Verification items for this drawing (mm, ordinates from the low corner). A direction names the side the tool comes from. Coordinates: 2 decimals unless noted, no trailing zeros. Order: outer loops, then holes, each group sorted by start corner. A loop starts at its lowest first (then second) coordinate and runs counter-clockwise, first axis right, second up. Notation, with made-up numbers: (55.25, 38.25) -> (59.25, 38.25) arc R4 cw to (59.25, 44.25) -> close; hole circle Ø11 at (-16, -31). An arc over 180 degrees is marked (long way). Write item = value, one per line. Start each with the question number.
1. Thickness scan on line 1 along Y through (x, z) = (13.97, 38.8); line 2 along Y through (x, z) = (13.5, 8); line 3 along X through (y, z) = (9, 4.5) (1 decimal). Record the ranges inside material, lowest first. Write a range as from..to.
2. Cross-section at A-A on x = 13.97. Record the cut outline in (y, z).
3. Set-up check for the marked faces 3 and 4: record each of +Z, -Z, +X, -X, +Y, -Y from which the full face is reachable in a straight line by a thin tool's end or side.
4. Cross-section at B-B on z = 36.5. Record the cut outline in (x, y).
5. Release check for a two-part mould opening along Y. For the marked faces 1 and 2 record: +Y half, -Y half, draft (parallel to the pull), parting line (faces both ways), or undercut.
6. Go/stop test with flat-tipped pins: P1, Ø5, axis at y = 3, z = 17, coming from the +X side; P2, Ø4, axis at x = 13, z = 22, coming from the +Y side; P3, Ø4, axis at x = 5, z = 17.5, coming from the +Y side. Record where each tip stops, or that it passes through.
7. Cross-section at C-C on z = 13. Record the cut outline in (x, y).
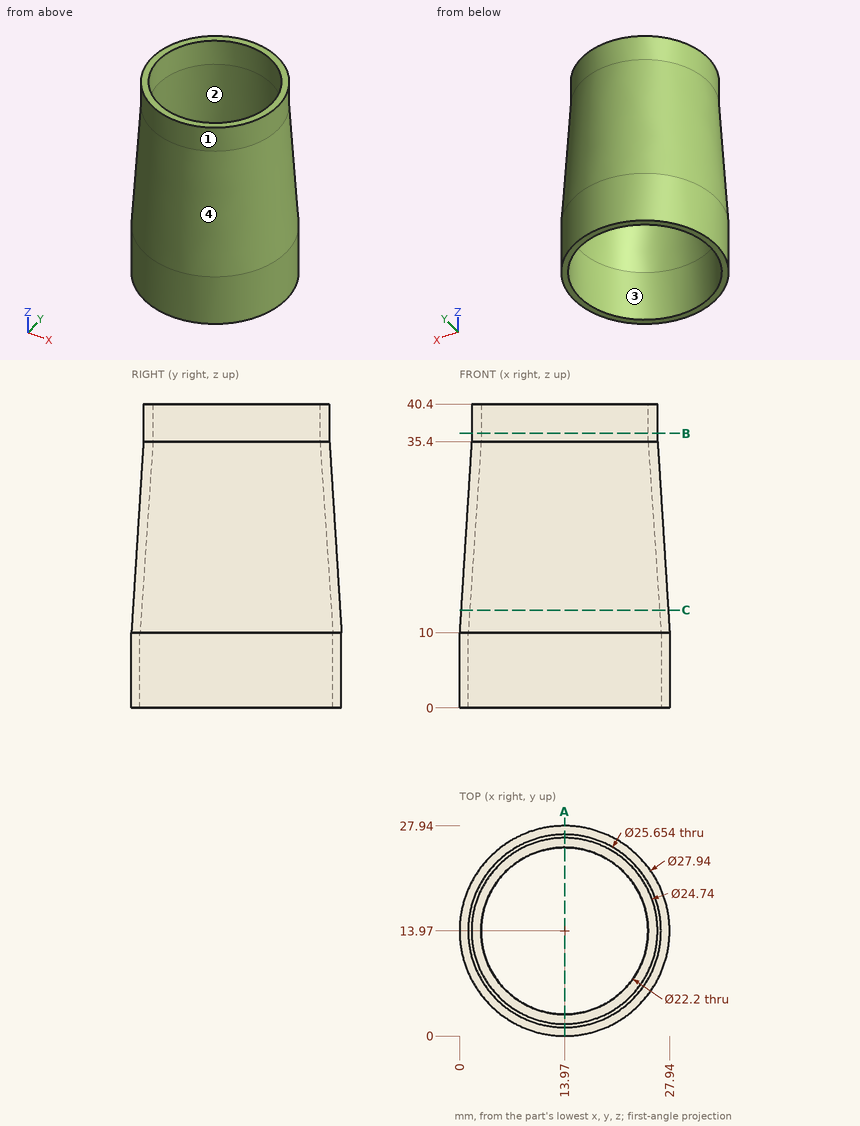
Worked out:
q1.line_1 = 1.6..2.87, 25.07..26.34
q1.line_2 = 0.01..1.15, 26.79..27.93
q1.line_3 = 0.9..2.1, 25.8..27
q2.outline = (0, 0) -> (1.14, 0) -> (1.14, 10) -> (2.87, 35.4) -> (2.87, 40.4) -> (1.6, 40.4) -> (1.6, 35.4) -> (0, 10) -> close; (25.07, 35.4) -> (26.8, 10) -> (26.8, 0) -> (27.94, 0) -> (27.94, 10) -> (26.34, 35.4) -> (26.34, 40.4) -> (25.07, 40.4) -> close
q3.face_3 = -Z
q3.face_4 = +Z
q4.outline = circle Ø24.74 at (13.97, 13.97); hole circle Ø22.2 at (13.97, 13.97)
q5.face_1 = parting line
q5.face_2 = undercut
q6.P1 = 24.53
q6.P2 = 27.3
q6.P3 = 25.54
q7.outline = circle Ø27.56 at (13.97, 13.97); hole circle Ø25.25 at (13.97, 13.97)
